Work out the finished part from the listing and answer in its coordinate system (mm). Face numbers are marked on the shaded views. A direction names the side the tool comes from. Round coordinates to 2 decimals unless told otherwise and drop trailing zeros. Order: outer loops, then holes, each group sorted by start corner. A loop starts at its lowest first (then second) coordinate and runs counter-clockwise, first axis right, second up. Notation, with made-up numbers: (75.25, -11.5) - (113.25, -11.5) arc R30 ccw to (113.25, 18.5) - close; hole circle Ø2 at (-27.75, 80). An arc over 180 degrees is marked (long way). Use CSV: the item, a comma, the result in double quotes.
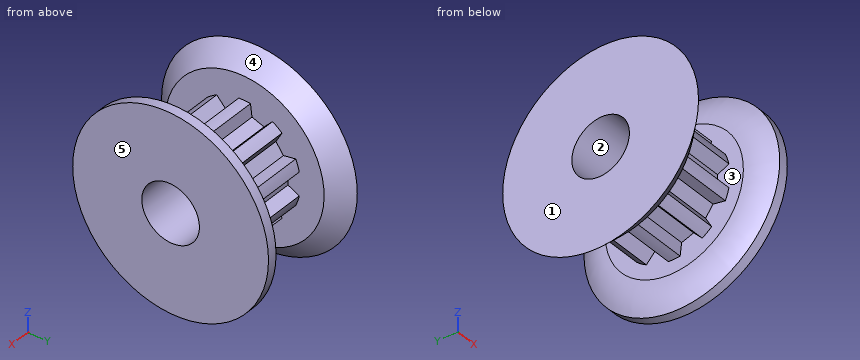
from build123d import *

# Parameters (mm, degrees)
SKETCH4_R          = 3.2385
SKETCH4_R_2        = 3.07975
CUT_EXTRUDE2_DEPTH = 4.064
CUT_EXTRUDE1_DEPTH = 4.064
CIRPATTERN1_COUNT  = 10


with BuildPart() as part:
    # Sketch1 → Revolve1 (revolve)
    with BuildSketch(Plane.XY, mode=Mode.PRIVATE) as revolve1_sk:
        with BuildLine():
            Line((-0.5588, 5.3975), (-0.5588, 1.5875))
            Line((-0.5588, 1.5875), (5.5626, 1.5875))
            Line((5.5626, 1.5875), (5.5626, 5.3975))
            Line((5.5626, 5.3975), (5.0419, 5.3975))
            ThreePointArc((5.0419, 5.3975), (4.654699632, 4.645356921), (4.5212, 3.81))
            Line((4.5212, 3.81), (4.5212, 3.2385))
            Line((4.5212, 3.2385), (0.4572, 3.2385))
            Line((0.4572, 3.2385), (0.4572, 4.3815))
            Line((0.4572, 4.3815), (-0.5588, 5.3975))
        make_face()
    revolve(revolve1_sk.sketch.rotate(Axis((-5.5626, 0, 0), (1, 0, 0)), 90), axis=Axis((-5.5626, 0, 0), (1, 0, 0)))

    # Sketch4 → Cut-Extrude2 (cut)
    with BuildSketch(Plane(origin=(0.4572, 0, 0), x_dir=(0, 0, -1), z_dir=(1, 0, 0))):
        Circle(SKETCH4_R)
        Circle(SKETCH4_R_2, mode=Mode.SUBTRACT)
    extrude(amount=CUT_EXTRUDE2_DEPTH, mode=Mode.SUBTRACT)

    # Sketch3 → Cut-Extrude1 (cut)
    with BuildSketch(Plane(origin=(0.4572, 0, 0), x_dir=(0, 0, -1), z_dir=(1, 0, 0))):
        with BuildLine():
            Line((-0.640454656, 3.012420604), (-0.349102168, 2.387613176))
            Line((-0.349102168, 2.387613176), (0.349102168, 2.387613176))
            Line((0.349102168, 2.387613176), (0.640454656, 3.012420604))
            ThreePointArc((0.640454656, 3.012420604), (0, 3.07975), (-0.640454656, 3.012420604))
        make_face()
    cut_extrude1 = extrude(amount=CUT_EXTRUDE1_DEPTH, mode=Mode.SUBTRACT)

    # CirPattern1: Cut-Extrude1 ×10 about axis
    cirpattern1_axis = Axis((0, 0, 0), (1, 0, 0))
    for i in range(1, CIRPATTERN1_COUNT):
        add(cut_extrude1.rotate(cirpattern1_axis, i * 360 / CIRPATTERN1_COUNT), mode=Mode.SUBTRACT)


solid = part.part
(1) Each of these flat-tipped pins is pushed along its axis until it touches: pin 1 (4 mm diameter, centred on y = -0.5, z = 0, fed in from -X); pin 2 (0.8 mm diameter, centred on x = 3, z = 0, fed in from -Y); pin 3 (2 mm diameter, centred on x = 2.5, z = -1.5, fed in from +Y). Where does it stop, or does it pass through?
Findings below:
pin 1,"stops at x = -0.56"
pin 2,"stops at y = -2.5"
pin 3,"stops at y = 3.01"
(2) The mould has two halves that part along X. Classify the marked faces 1, 2 and 3: released by +X, released by -X, zero draft, split by the parting line, or undercut.
Findings below:
face 1,"released by -X"
face 2,"zero draft"
face 3,"undercut"
(3) Find section B-B (y = 0). Determine the outline of the cut face in (x, z), and give its area (3 significant figures).
Findings below:
outline,"(-0.56, -5.4) - (0.46, -4.38) - (0.46, -3.08) - (4.52, -3.08) - (4.52, -3.81) arc R2.68 ccw to (5.04, -5.4) - (5.56, -5.4) - (5.56, -1.59) - (-0.56, -1.59) - close; (-0.56, 1.59) - (5.56, 1.59) - (5.56, 5.4) - (5.04, 5.4) arc R2.68 ccw to (4.52, 3.81) - (4.52, 3.08) - (0.46, 3.08) - (0.46, 4.38) - (-0.56, 5.4) - close"
area,"26.2 mm²"
(4) For the marked faces 4 and 5, determine the directions among +Z, -Z, +X, -X, +Y, -Y from which every point of the face is accessible in a straight line to the end or side of a thin tool.
Findings below:
face 4,"none"
face 5,"+Z, -Z, +X, +Y, -Y"
(5) Find the intervals of material crossed by L1, parallel to Y at x = 1, z = 0; L2, parallel to X at y = -3, z = -2.25; L3, parallel to Y at x = 3, z = 2.5, in increasing order. Write a range as from..to.
Findings below:
L1,"y = -2.39..-1.59, 1.59..2.39"
L2,"x = -0.56..0.46, 4.52..5.56"
L3,"y = -1.8..-1.38, -0.39..0.39, 1.38..1.8"
(6) Find section A-A (z = 0). Determine the outline of the cut face in (x, y), and give its area (3 significant figures).
Findings below:
outline,"(-0.56, -5.4) - (0.46, -4.38) - (0.46, -2.39) - (4.52, -2.39) - (4.52, -3.81) arc R2.68 ccw to (5.04, -5.4) - (5.56, -5.4) - (5.56, -1.59) - (-0.56, -1.59) - close; (-0.56, 1.59) - (5.56, 1.59) - (5.56, 5.4) - (5.04, 5.4) arc R2.68 ccw to (4.52, 3.81) - (4.52, 2.39) - (0.46, 2.39) - (0.46, 4.38) - (-0.56, 5.4) - close"
area,"20.6 mm²"
